Check sheet for the modelled part. Datum: model origin and axes. Units: mm. Face numbers are marked on the shaded views. A direction names the side the tool comes from. Coordinates: 2 decimals unless noted, no trailing zeros. Write each loop counter-clockwise with the first axis right and the second up, starting at its lowest first coordinate (ties: lowest second). Pieces come first, ordered by that corner, then holes. Notation, with made-up numbers: M -18.5,45.25 L 21.5,45.25 A17 cw 21.5,49.25 Z; hole C 4,-7 d9. An arc over 180 degrees is marked long. Answer as CSV lines item,"result". Start each with the question number.
Q1. Sectioned sample at D-D, the plane y = 2.5. Record the cut outline in (x, z), then the cut area to 3 significant figures.
Q2. Mould release check, pull along Y, two halves, no side actions. Record for the marked faces 1, 2, 3 and 4: pulls with the +Y half, pulls with the -Y half, needs draft (parallel to the pull), parting line crosses it, or undercut.
Q3. Access from +Z, -Z, +X, -X, +Y, -Y to the whole of each face (thin tool, end or side, straight path). Record for the marked faces 5, 6, 7 and 8.
Q4. Thickness scan on line 1 along Y through (x, z) = (-8.1, 1.4); line 2 along Z through (x, y) = (4, -2.75); line 3 along Z through (x, y) = (6.5, 0.25). Record the ranges inside material, lowest first. Write a range as from..to.
Q5. Sectioned sample at A-A, the plane x = -8.1. Record the cut outline in (y, z).
Q6. Sectioned sample at C-C, the plane x = 2.75. Record the cut outline in (y, z), then the cut area to 3 significant figures.
Q7. Depth check by flat-ended pin: pin 1 Ø1 at (y, z) = (-3, 3) entering from -X; pin 2 Ø4 at (x, y) = (8.1, 0) entering from -Z; pin 3 Ø6 at (x, y) = (7.5, 4) entering from +Z; pin 4 Ø1.6 at (x, z) = (-1, -1.5) entering from -Y. Enter the tip coordinate at first touch or a pass-through.
Q8. Sectioned sample at B-B, the plane y = 0. Record the cut outline in (x, z), then the cut area to 3 significant figures.
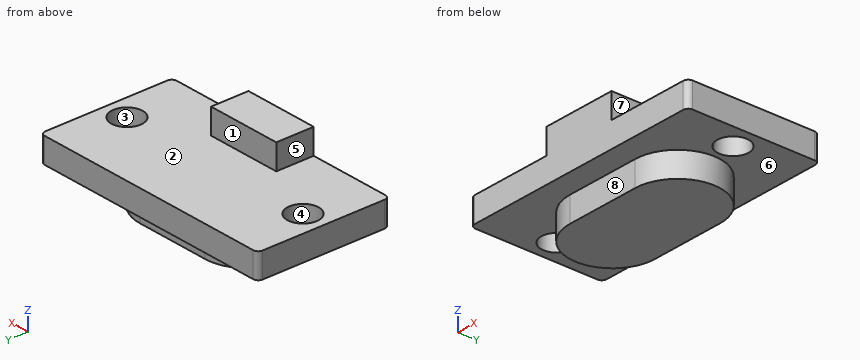
from build123d import *

# Parameters (mm, degrees)
SKETCH_1_W      = 20
SKETCH_1_H      = 10.6
SKETCH_1_R      = 1.25
EXTRUDE_1_DEPTH = 2
EXTRUDE_2_DEPTH = 2
SKETCH_3_W      = 6
SKETCH_3_H      = 3
EXTRUDE_3_DEPTH = 2
FILLET_1_R      = 0.4


with BuildPart() as part:
    # 草图1 → 凸台-拉伸1 (new body)
    with BuildSketch(Plane.XY):
        Rectangle(SKETCH_1_W, SKETCH_1_H)
        with Locations((8.1, 0)):
            Circle(SKETCH_1_R, mode=Mode.SUBTRACT)
        with Locations(Location((-8.1, 0, 0), (0, 0, 180))):
            Circle(SKETCH_1_R, mode=Mode.SUBTRACT)
    extrude(amount=EXTRUDE_1_DEPTH)

    # 草图2 → 凸台-拉伸2 (add)
    with BuildSketch(Plane(origin=(0, 0, 0), x_dir=(-1, 0, 0), z_dir=(0, 0, -1))):
        with BuildLine():
            Line((-3, 3.4), (3, 3.4))
            ThreePointArc((3, 3.4), (6.4, 0), (3, -3.4))
            Line((3, -3.4), (-3, -3.4))
            ThreePointArc((-3, -3.4), (-6.4, 0), (-3, 3.4))
        make_face()
    extrude(amount=EXTRUDE_2_DEPTH)

    # 草图3 → 凸台-拉伸3 (add)
    with BuildSketch(Plane.XY.offset(2)):
        with Locations((0, -3.8)):
            Rectangle(SKETCH_3_W, SKETCH_3_H)
    extrude(amount=EXTRUDE_3_DEPTH)

    # 圆角1
    fillet_1_edges = [part.edges().sort_by_distance(p)[0] for p in [
        (10, -5.3, 1),
        (-10, -5.3, 1),
        (-10, 5.3, 1),
        (10, 5.3, 1),
    ]]
    fillet(fillet_1_edges, radius=FILLET_1_R)


solid = part.part
Output:
1,outline,"M -10,0 L -5.3,0 L -5.3,-2 L 5.3,-2 L 5.3,0 L 10,0 L 10,2 L -10,2 Z"
1,area,"61.2 mm^2"
2,face 1,"pulls with the +Y half"
2,face 2,"needs draft"
2,face 3,"undercut"
2,face 4,"undercut"
3,face 5,"+Z, -X, +Y, -Y"
3,face 6,"-Z"
3,face 7,"+Z, +X, +Y, -Y"
3,face 8,"-Z, +X, -X, -Y"
4,line 1,"y = -5.3..-1.25, 1.25..5.3"
4,line 2,"z = -2..2"
4,line 3,"z = 0..2"
5,outline,"M -5.3,0 L -1.25,0 L -1.25,2 L -5.3,2 Z; M 1.25,0 L 5.3,0 L 5.3,2 L 1.25,2 Z"
6,outline,"M -5.3,0 L -3.4,0 L -3.4,-2 L 3.4,-2 L 3.4,0 L 5.3,0 L 5.3,2 L -2.3,2 L -2.3,4 L -5.3,4 Z"
6,area,"40.8 mm^2"
7,pin 1,"stops at x = -3"
7,pin 2,"stops at z = -2"
7,pin 3,"stops at z = 2"
7,pin 4,"stops at y = -3.4"
8,outline,"M -10,0 L -9.35,0 L -9.35,2 L -10,2 Z; M -6.85,0 L -6.4,0 L -6.4,-2 L 6.4,-2 L 6.4,0 L 6.85,0 L 6.85,2 L -6.85,2 Z; M 9.35,0 L 10,0 L 10,2 L 9.35,2 Z"
8,area,"55.6 mm^2"
